For this review, take the finished solid that the model builds, in its own axes (mm). Coordinates: 2 decimals unless noted, no trailing zeros. Order: outer loops, then holes, each group sorted by start corner. A loop starts at its lowest first (then second) coordinate and runs counter-clockwise, first axis right, second up.
from build123d import *

# Parameters (mm, degrees)
ESQUISSE2_W        = 2000
ESQUISSE2_H        = 2000
BOSS_EXTRU_2_DEPTH = 10
ESQUISSE1_R        = 110
BOSS_EXTRU_6_DEPTH = 1


with BuildPart() as part:
    # Esquisse2 → Boss.-Extru.2 (new body)
    with BuildSketch(Plane(origin=(0, 0, 0), x_dir=(1, 0, 0), z_dir=(0, 1, 0))):
        Rectangle(ESQUISSE2_W, ESQUISSE2_H)
    extrude(amount=-BOSS_EXTRU_2_DEPTH)

    # Esquisse1 → Boss.-Extru.6 (add)
    with BuildSketch(Plane(origin=(0, 0, 0), x_dir=(1, 0, 0), z_dir=(0, 1, 0))):
        with Locations(Location((-140, 465, 0), (0, 0, 90))):
            Circle(ESQUISSE1_R)
        with BuildLine():
            Line((-30, -100), (-450, -100))
            ThreePointArc((-450, -100), (-534.852813742, -135.147186258), (-570, -220))
            Line((-570, -220), (-570, -700))
            ThreePointArc((-570, -700), (-575.857864376, -714.142135624), (-590, -720))
            Line((-590, -720), (-660, -720))
            ThreePointArc((-660, -720), (-674.142135624, -714.142135624), (-680, -700))
            Line((-680, -700), (-680, 700))
            ThreePointArc((-680, 700), (-674.142135624, 714.142135624), (-660, 720))
            Line((-660, 720), (-649.834574491, 720))
            ThreePointArc((-649.834574491, 720), (-643.12759549, 718.841879754), (-637.197365306, 715.501643268))
            Line((-637.197365306, 715.501643268), (-497.957421247, 601.990819307))
            ThreePointArc((-497.957421247, 601.990819307), (-491.401573638, 592.112926645), (-491.58977759, 580.258961883))
            ThreePointArc((-491.58977759, 580.258961883), (-264.079111523, 116.425224545), (205.33854603, 332.179487179))
            ThreePointArc((205.33854603, 332.179487179), (212.682724123, 341.486202467), (224.005494464, 345))
            Line((224.005494464, 345), (480, 345))
            ThreePointArc((480, 345), (564.852813742, 380.147186258), (600, 465))
            Line((600, 465), (600, 685))
            ThreePointArc((600, 685), (605.857864376, 699.142135624), (620, 705))
            Line((620, 705), (700, 705))
            ThreePointArc((700, 705), (714.142135624, 699.142135624), (720, 685))
            Line((720, 685), (720, 0))
            Line((720, 0), (710, 0))
            Line((710, 0), (710, 675))
            ThreePointArc((710, 675), (704.142135624, 689.142135624), (690, 695))
            Line((690, 695), (630, 695))
            ThreePointArc((630, 695), (615.857864376, 689.142135624), (610, 675))
            Line((610, 675), (610, 455))
            ThreePointArc((610, 455), (574.852813742, 370.147186258), (490, 335))
            Line((490, 335), (230.809924355, 335))
            ThreePointArc((230.809924355, 335), (219.629584467, 331.583123952), (212.269428137, 322.5))
            ThreePointArc((212.269428137, 322.5), (-267.432601024, 107.004284668), (-503.077865902, 577.135914371))
            ThreePointArc((-503.077865902, 577.135914371), (-503.043324922, 588.826673493), (-509.55001808, 598.539447869))
            Line((-509.55001808, 598.539447869), (-646.274962028, 710))
            Line((-646.274962028, 710), (-650, 710))
            ThreePointArc((-650, 710), (-664.142135624, 704.142135624), (-670, 690))
            Line((-670, 690), (-670, -690))
            ThreePointArc((-670, -690), (-664.142135624, -704.142135624), (-650, -710))
            Line((-650, -710), (-600, -710))
            ThreePointArc((-600, -710), (-585.857864376, -704.142135624), (-580, -690))
            Line((-580, -690), (-580, -210))
            ThreePointArc((-580, -210), (-544.852813742, -125.147186258), (-460, -90))
            Line((-460, -90), (-30, -90))
            Line((-30, -90), (-30, -100))
        make_face()
        with BuildLine():
            Line((-30, -340), (-310, -340))
            ThreePointArc((-310, -340), (-324.142135624, -345.857864376), (-330, -360))
            Line((-330, -360), (-330, -840))
            ThreePointArc((-330, -840), (-365.147186258, -924.852813742), (-450, -960))
            Line((-450, -960), (-855, -960))
            ThreePointArc((-855, -960), (-939.852813742, -924.852813742), (-975, -840))
            Line((-975, -840), (-975, 840))
            ThreePointArc((-975, 840), (-939.852813742, 924.852813742), (-855, 960))
            Line((-855, 960), (-600, 960))
            ThreePointArc((-600, 960), (-559.758125993, 953.051278526), (-524.176744886, 933.009859606))
            Line((-524.176744886, 933.009859606), (-346.310911019, 788.010538519))
            ThreePointArc((-346.310911019, 788.010538519), (-335.314603965, 783.579609444), (-323.741717124, 786.152582721))
            ThreePointArc((-323.741717124, 786.152582721), (-15.920888477, 813.574775455), (205.33854603, 597.820512821))
            ThreePointArc((205.33854603, 597.820512821), (212.682724123, 588.513797533), (224.005494464, 585))
            Line((224.005494464, 585), (340, 585))
            ThreePointArc((340, 585), (354.142135624, 590.857864376), (360, 605))
            Line((360, 605), (360, 825))
            ThreePointArc((360, 825), (395.147186258, 909.852813742), (480, 945))
            Line((480, 945), (840, 945))
            ThreePointArc((840, 945), (924.852813742, 909.852813742), (960, 825))
            Line((960, 825), (960, 0))
            Line((960, 0), (970, 0))
            Line((970, 0), (970, 835))
            ThreePointArc((970, 835), (934.852813742, 919.852813742), (850, 955))
            Line((850, 955), (470, 955))
            ThreePointArc((470, 955), (385.147186258, 919.852813742), (350, 835))
            Line((350, 835), (350, 615))
            ThreePointArc((350, 615), (344.142135624, 600.857864376), (330, 595))
            Line((330, 595), (230.809924355, 595))
            ThreePointArc((230.809924355, 595), (219.629584467, 598.416876048), (212.269428137, 607.5))
            ThreePointArc((212.269428137, 607.5), (-12.567398976, 822.995715332), (-322.997635007, 798.034330936))
            ThreePointArc((-322.997635007, 798.034330936), (-334.44162777, 795.644755332), (-345.266298667, 800.060810349))
            Line((-345.266298667, 800.060810349), (-520.617132423, 943.009859606))
            ThreePointArc((-520.617132423, 943.009859606), (-556.198513529, 963.051278526), (-596.440387536, 970))
            Line((-596.440387536, 970), (-865, 970))
            ThreePointArc((-865, 970), (-949.852813742, 934.852813742), (-985, 850))
            Line((-985, 850), (-985, -850))
            ThreePointArc((-985, -850), (-949.852813742, -934.852813742), (-865, -970))
            Line((-865, -970), (-440, -970))
            ThreePointArc((-440, -970), (-355.147186258, -934.852813742), (-320, -850))
            Line((-320, -850), (-320, -370))
            ThreePointArc((-320, -370), (-314.142135624, -355.857864376), (-300, -350))
            Line((-300, -350), (-30, -350))
            Line((-30, -350), (-30, -340))
        make_face()
    extrude(amount=BOSS_EXTRU_6_DEPTH)


solid = part.part
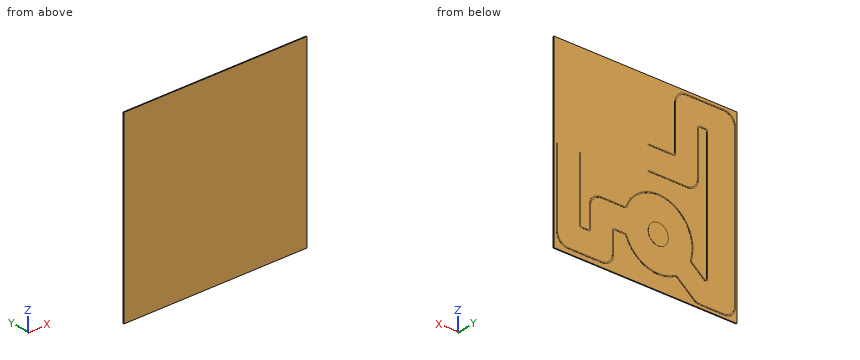
1. Take a section at C-C, the plane x = -384. Give the boundary of the cut face in (y, z), plus the area to 3 significant figures.
Answer below:
outline: (-10, -1000) - (0, -1000) - (0, -831.64) - (1, -831.64) - (1, -818.74) - (0, -818.74) - (0, -186.86) - (1, -186.86) - (1, -173.69) - (0, -173.69) - (0, 90) - (1, 90) - (1, 100) - (0, 100) - (0, 940.22) - (1, 940.22) - (1, 956.13) - (0, 956.13) - (0, 1000) - (-10, 1000) - close
area: 20,100 mm2
2. To check wall thickness, follow L1, parallel to Y at x = -49.5, z = -190.5. State the ranges of the line that lie inside material, in increasing order.
Answer below:
L1: y = -10 to 0
3. Clearance check with flat-ended pins moving along their axes: pin 1 Ø0.8 at (x, y) = (-275.5, 0.5) entering from -Z; pin 2 Ø0.5 at (y, z) = (0.5, -731.5) entering from +X; pin 3 Ø0.8 at (x, y) = (395, 0.5) entering from -Z. State where each tip first meets the part, or that it passes through.
Answer below:
pin 1: stops at z = -820.17
pin 2: stops at x = 970
pin 3: stops at z = -928.99
4. Take a section at A-A, the plane x = -140. Give the boundary of the cut face in (y, z).
Answer below:
outline: (-10, -1000) - (0, -1000) - (0, -845) - (1, -845) - (1, -835) - (0, -835) - (0, -575) - (1, -575) - (1, -355) - (0, -355) - (0, -95) - (1, -95) - (1, -85) - (0, -85) - (0, 90) - (1, 90) - (1, 100) - (0, 100) - (0, 340) - (1, 340) - (1, 350) - (0, 350) - (0, 1000) - (-10, 1000) - close
